Autodesk Inventor part; units mm, degrees
ref_plane "YZ Plane" through (0, 0, 0) normal (1, 0, 0) x (0, 1, 0)
ref_plane "XZ Plane" through (0, 0, 0) normal (0, 1, 0) x (-1, 0, 0)
ref_plane "XY Plane" through (0, 0, 0) normal (0, 0, 1) x (1, 0, 0)
sketch "草圖1" plane through (0, 0, 0) normal (0, 0, 1) x (1, 0, 0)
  line L0 (0, 0) -> (115, 0)
  line L1 (0, 0) -> (-450, 0)
  line L2 (-167.5, 95) -> (135, 95)
  line L3 (-167.5, 95) -> (-470, 95)
  line L4 (-167.5, 20) -> (95, 20)
  line L5 (-167.5, 20) -> (-430, 20)
  line L6 (-430, 20) -> (-470, 95)
  line L7 (95, 20) -> (135, 95)
  line L8 (115, 0) -> (165.6667, 95)
  line L9 (165.6667, 95) -> (210.6667, 95)
  line L10 (210.6667, 95) -> (210.6667, 115)
  line L11 (210.6667, 115) -> (-559.3333, 115)
  line L12 (-450, 0) -> (-500.6667, 95)
  line L13 (-500.6667, 95) -> (-545.6667, 95)
  line L14 (-545.6667, 95) -> (-545.6667, 115)
  line L15 (-130, 20) -> (-130, 95)
  line L16 (-130, 20) -> (-150, 20)
  line L17 (-150, 20) -> (-150, 95)
  dimension "d0" = 115
  dimension "d2" = 450
  dimension "d5" = 302.5
  dimension "d6" = 302.5
  dimension "d8" = 262.5
  dimension "d9" = 262.5
  dimension "d10" = 45
  dimension "d11" = 20
  dimension "d13" = 770
  dimension "d14" = 45
  dimension "d16" = 20
extrude "擠出1" add sketch "草圖1" along normal blind 20 contours L1 L12 L13 L14 L11 L10 L9 L8 L0 | L2 L15 L4 L17
sketch "草圖2" plane through (-545.6667, 115, 0) normal (0, 1, 0) x (1, 0, 0)
  line L0 (756.3333, 0) -> (756.3333, -20)
  circle A0 centre (723.8333, -10) radius 5
  line L1 (0, 0) -> (0, -20)
  circle A1 centre (32.5, -10) radius 5
  point P0 (545.6667, 0)
  dimension "d21" = 10
  dimension "d23" = 10
extrude "擠出2" add sketch "草圖2" along normal blind 20
sketch "草圖3" plane through (-513.1667, 135, 10) normal (0, 1, 0) x (1, 0, 0)
  circle A0 centre (0, 0) radius 5
  circle A1 centre (0, 0) radius 17.5
  point P0 (513.1667, 10)
  dimension "d26" = 35
extrude "擠出3" add sketch "草圖3" along normal blind 10 contours A0 | A1
sketch "草圖4" plane through (178.1667, 135, 10) normal (0, 1, 0) x (1, 0, 0)
  circle A0 centre (0, 0) radius 17.5
  point P0 (-178.1667, 10)
  dimension "d29" = 35
extrude "擠出4" add sketch "草圖4" along normal blind 10
properties part number "DOF7"
Input: part model. Units: mm. Frame: model coordinates. A direction names the side the tool comes from. Coordinates: 2 decimals unless noted, no trailing zeros. Order: outer loops, then holes, each group sorted by start corner. A loop starts at its lowest first (then second) coordinate and runs counter-clockwise, first axis right, second up. Notation, with made-up numbers: M -4,-13 L 21,-13 A27 ccw 21,7 Z; hole C 62,21.25 d6. An arc over 180 degrees is marked long. One line per question, with ' | ' between items.
Item 1: Section A-A (x = -443.5). Output: boundary loops of the cut face in (y, z), then the cut area to 3 significant figures.
Geometry results:
outline: M 0,0 L 45.31,0 L 45.31,20 L 0,20 Z; M 95,0 L 115,0 L 115,20 L 95,20 Z | area: 1,310 mm^2
Item 2: Ray query, line 1 along X through (y, z) = (73.5, 7); line 2 along Y through (x, z) = (-415, 13); line 3 along X through (y, z) = (91, 17.5). Return the intervals inside material, ascending.
Geometry results:
line 1: x = -489.2 to -458.53, -150 to -130, 123.53 to 154.2 | line 2: y = 0 to 20, 95 to 115 | line 3: x = -498.53 to -467.87, -150 to -130, 132.87 to 163.53
Item 3: Section B-B (y = 13.5). Output: boundary loops of the cut face in (x, z), then the cut area to 3 significant figures.
Geometry results:
outline: M -457.2,0 L 122.2,0 L 122.2,20 L -457.2,20 Z | area: 11,600 mm^2
Item 4: Reachability of faces 5 (the cylindrical face through (160.684, 139.93, 10.769)), 6 (the flat face through (188, 95, 10)), 7 (the flat face through (-150, 57, 10)), 8 (the flat face through (182, 135, 14)) from +Z, -Z, +X, -X, +Y, -Y: full face, straight path, thin tool, end or side. Return the list, or none.
Geometry results:
face 5: +Y | face 6: +Z, -Z, +X, -Y | face 7: +Z, -Z | face 8: none
Item 5: Draft query along X for faces 1 (the flat face through (139.98, 46.84, 9.86)), 2 (the flat face through (-474.98, 46.84, 9.86)), 3 (the flat face through (178, 145, 10)), 4 (the flat face through (114.72, 56.975, 9.86)). Return one class per face: released by +X, released by -X, zero draft, split by the parting line, or undercut.
Geometry results:
face 1: released by +X | face 2: released by -X | face 3: zero draft | face 4: undercut
Item 6: Pin query (flat end, axial travel): pin 1 (1 mm diameter, centred on x = 34, y = 18.5, fed in from +Z); pin 2 (3 mm diameter, centred on y = 20, z = 16.5, fed in from -X); pin 3 (5 mm diameter, centred on x = -9, z = 13.5, fed in from +Y). Return the tip coordinate at first contact, or that it passes through.
Geometry results:
pin 1: stops at z = 20 | pin 2: stops at x = -461.47 | pin 3: stops at y = 115
